Can you work these out from the model? Positions are in its coordinate system, mm. A direction names the side the tool comes from. Round coordinates to 2 decimals unless told otherwise and drop trailing zeros. Loops run counter-clockwise (first coordinate to the right, second up) from the corner with the lowest first, then second, coordinate; pieces in that order, holes last.
Autodesk Inventor part; units mm, degrees
ref_plane "YZ Plane" through (0, 0, 0) normal (1, 0, 0) x (0, 1, 0)
ref_plane "XZ Plane" through (0, 0, 0) normal (0, 1, 0) x (-1, 0, 0)
ref_plane "XY Plane" through (0, 0, 0) normal (0, 0, 1) x (1, 0, 0)
sketch "Sketch1" plane through (0, 0, 0) normal (0, 1, 0) x (-1, 0, 0)
  line L0 (0, -6) -> (0, 0)
  circle A0 centre (-20, -3) radius 1.5
  circle A1 centre (-38, -3) radius 1.5
  circle A2 centre (0, -3) radius 1.5
  circle A3 centre (0, -3) radius 3
  circle A4 centre (-38, -3) radius 3
  line L1 (-38, 0) -> (0, 0)
  line L2 (0, -6) -> (-38, -6)
  point P0 (0, -4.5)
  point P1 (0, -1.5)
  dimension "d11" = 3
  dimension "d26" = 3
  dimension "d27" = 3
  dimension "d28" = 6
  dimension "d29" = 6
extrude "Extrusion2" add sketch "Sketch1" along normal blind 15 contours A0
ref_plane "Work Plane1" through (0, 1, 0) normal (0, 1, 0) x (1, 0, 0)
sketch "Sketch2" plane through (0, 1, 0) normal (0, 1, 0) x (1, 0, 0)
  circle A0 centre (20, 3) radius 1.5
  circle A1 centre (20, 3) radius 2.5
  circle A2 centre (20, 3) radius 1.5
  point P0 (0, 0)
  dimension "d14" = 5
extrude "Extrusion3" add sketch "Sketch2" along normal blind 3
chamfer "Chamfer1" distance 0.5 angle 45 1 edges at (21.5, 15, -3)
extrude "Extrusion4" add sketch "Sketch1" along normal blind 1 contours A3 L0 A2 | L2 A4 L1 A3 | L0 A2 A3 | A4
thread "Thread2"
properties part number "linkToActuator3"
(1) For faces 1 (the cylindrical face through (-3, 0.5, -2.9)), 2 (the cylindrical face through (17.5, 2.5, -2.9)), which set-ups out of +Z, -Z, +X, -X, +Y, -Y let a thin tool reach every point of the face, with its end or its side?
Worked answers:
face 1: -X, +Y, -Y
face 2: +Y
(2) If we section it at C-C, the plane y = 6.75: List the corners of the cut face in (x, z) for me.
Worked answers:
outline: circle Ø3 at (20, -3)
(3) If we section it at B-B, the plane x = 20: List the corners of the cut face in (y, z) for me.
Worked answers:
outline: (0, -6) - (1, -6) - (1, -5.5) - (4, -5.5) - (4, -4.5) - (14.5, -4.5) - (15, -4) - (15, -2) - (14.5, -1.5) - (4, -1.5) - (4, -0.5) - (1, -0.5) - (1, 0) - (0, 0) - close
(4) If we section it at A-A, the plane z = -3: List the corners of the cut face in (x, y) for me.
Worked answers:
outline: (-3, 0) - (-1.5, 0) - (-1.5, 1) - (-3, 1) - close; (1.5, 0) - (36.5, 0) - (36.5, 1) - (22.5, 1) - (22.5, 4) - (21.5, 4) - (21.5, 14.5) - (21, 15) - (19, 15) - (18.5, 14.5) - (18.5, 4) - (17.5, 4) - (17.5, 1) - (1.5, 1) - close; (39.5, 0) - (41, 0) - (41, 1) - (39.5, 1) - close
(5) If I drill on line 1 (Z direction, x = 38, y = 0.5); line 2 (Y direction, x = 34, z = -2.65); line 3 (X direction, y = 8, z = -2.95), over which ranges is the centre line in solid material (lowest first)?
Worked answers:
line 1: z = -6 to -4.5, -1.5 to 0
line 2: y = 0 to 1
line 3: x = 18.5 to 21.5
(6) Will these pins go through, and if not, where does the flat tip stop? P1, Ø1, axis at x = 16, z = -4.5, coming from the -Y side; P2, Ø2, axis at y = 1.5, z = -5, coming from the -X side; P3, Ø8, axis at x = 22.5, y = 10, coming from the +Z side; P4, Ø1.8, axis at x = 26, z = -2, coming from the +Y side.
Worked answers:
P1: stops at y = 0
P2: stops at x = -2.78
P3: stops at z = -1.5
P4: stops at y = 1
(7) If we mould it in two halves opening along Z, with no side actions, what happens to faces 3 (the flat face through (20, 4, -1)), 4 (the cylindrical face through (0.325, 0.493, -1.536)), 5 (the cylindrical face through (21.5, 9.18, -3.07))? For each: released by +Z, released by -Z, zero draft, split by the parting line, or undercut.
Worked answers:
face 3: zero draft
face 4: undercut
face 5: split by the parting line
(8) If we section it at D-D, the plane z = -4.9: List the corners of the cut face in (x, y) for me.
Worked answers:
outline: (-2.32, 0) - (40.32, 0) - (40.32, 1) - (21.62, 1) - (21.62, 4) - (18.38, 4) - (18.38, 1) - (-2.32, 1) - close
